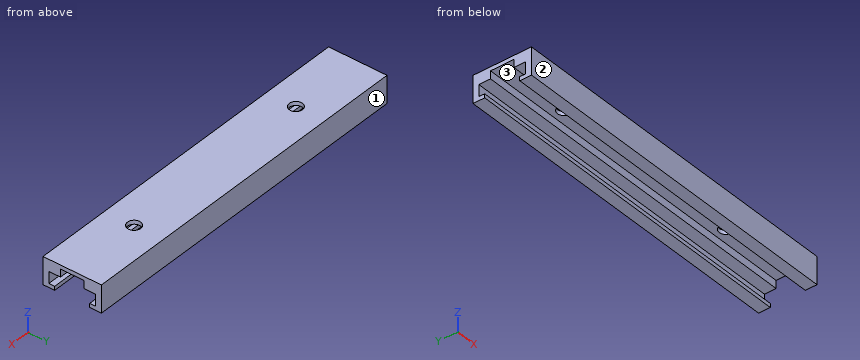
Autodesk Inventor part; units mm, degrees
ref_plane "YZ Plane" through (0, 0, 0) normal (1, 0, 0) x (0, 1, 0)
ref_plane "XZ Plane" through (0, 0, 0) normal (0, 1, 0) x (-1, 0, 0)
ref_plane "XY Plane" through (0, 0, 0) normal (0, 0, 1) x (1, 0, 0)
sketch "スケッチ1" plane through (0, 0, 0) normal (1, 0, 0) x (0, 1, 0)
  line L0 (0, 0) -> (15, 0)
  line L1 (15, 0) -> (15, -7)
  line L2 (0, -7) -> (0, 0)
  line L3 (7.5, 0) -> (7.5, -7)
  line L4 (7.5, -1) -> (10.5, -1)
  line L5 (10.5, -1) -> (10.5, -3)
  line L6 (10.5, -3) -> (13.5, -3)
  line L7 (13.5, -3) -> (13.5, -6)
  line L8 (13.5, -6) -> (12, -6)
  line L9 (12, -6) -> (12, -7)
  line L10 (7.5, -1) -> (4.5, -1)
  line L11 (4.5, -1) -> (4.5, -3)
  line L12 (4.5, -3) -> (1.5, -3)
  line L13 (1.5, -3) -> (1.5, -6)
  line L14 (1.5, -6) -> (3, -6)
  line L15 (3, -6) -> (3, -7)
  line L16 (15, -7) -> (12, -7)
  line L17 (3, -7) -> (0, -7)
  dimension "d0" = 15
  dimension "d1" = 7
  dimension "d2" = 3
  dimension "d3" = 2
  dimension "d5" = 3
  dimension "d6" = 3
  dimension "d7" = 1.5
  dimension "d9" = 1
extrude "押し出し1" add sketch "スケッチ1" along normal blind 90
sketch "スケッチ2" plane through (0, 0, 0) normal (0, 0, 1) x (1, 0, 0)
  line L0 (0, 4.5) -> (0, 10.5)
  line L1 (0, 7.5) -> (90, 7.5)
  line L2 (90, 4.5) -> (90, 10.5)
  line L3 (0, 15) -> (0, 0)
  line L4 (90, 15) -> (90, 0)
  point P0 (19.5, 7.5)
  point P1 (70.5, 7.5)
  dimension "d12" = 19.5
  dimension "d20" = 19.5
hole "穴1" at (19.5, 7.5, 0) at (70.5, 7.5, 0) direction (0, 0, -1) diameter 3.4 end through all
properties part number "slider2a2" material "アルミニウム 6061-AHC"
Could you check a few things on this model? Use its own coordinates, in mm. Face numbers are marked on the shaded views. Give positions to 0.01 mm unless a question says otherwise; leave off trailing zeros. Order: outer loops, then holes, each group sorted by start corner. A loop starts at its lowest first (then second) coordinate and runs counter-clockwise, first axis right, second up. Notation, with made-up numbers: (-17.5, 38.25) - (19.5, 38.25) arc R22 cw to (19.5, 51.25) - close; hole circle Ø5 at (18, -0.5). An arc over 180 degrees is marked (long way). One line per item, written item: value. Start each with the question number.
1. Imagine slicing it at C-C on z = -5.25. List the corners of the cut face in (x, y) for me, plus the area to 3 significant figures.
2. Imagine slicing it at A-A on x = 70.5. List the corners of the cut face in (y, z) for me, plus the area to 3 significant figures.
3. Imagine slicing it at D-D on x = 14.5. List the corners of the cut face in (y, z) for me, plus the area to 3 significant figures.
4. For P1, Ø0.6, axis at x = 51, z = -2.5, coming from the -Y side, with a flat end and sliding along its axis, tell me the tip position at first contact or that it passes through.
5. If I drill on probe 1 along X at (y, z) = (7.5, -0.5); probe 2 along Y at (x, z) = (70, -2.5); probe 3 along Z at (x, y) = (59.5, 13.25), over which ranges is the centre line in solid material (lowest first)?
6. Imagine slicing it at B-B on y = 7.5. List the corners of the cut face in (x, z) for me, plus the area to 3 significant figures.
7. Thinking about a two-plate mould opening in Y: for the marked faces 1, 2 and 3, which applies, +Y half, -Y half, draft (parallel to the pull), parting line (faces both ways), or undercut?
Values:
1. outline: (0, 0) - (90, 0) - (90, 1.5) - (0, 1.5) - close; (0, 13.5) - (90, 13.5) - (90, 15) - (0, 15) - close
1. area: 270 mm²
2. outline: (0, -7) - (3, -7) - (3, -6) - (1.5, -6) - (1.5, -3) - (4.5, -3) - (4.5, -1) - (5.8, -1) - (5.8, 0) - (0, 0) - close; (9.2, -1) - (10.5, -1) - (10.5, -3) - (13.5, -3) - (13.5, -6) - (12, -6) - (12, -7) - (15, -7) - (15, 0) - (9.2, 0) - close
2. area: 44.6 mm²
3. outline: (0, -7) - (3, -7) - (3, -6) - (1.5, -6) - (1.5, -3) - (4.5, -3) - (4.5, -1) - (10.5, -1) - (10.5, -3) - (13.5, -3) - (13.5, -6) - (12, -6) - (12, -7) - (15, -7) - (15, 0) - (0, 0) - close
3. area: 48.0 mm²
4. P1: y = 0
5. probe 1: 0 to 17.8, 21.2 to 68.8, 72.2 to 90
5. probe 2: 0 to 4.5, 10.5 to 15
5. probe 3: -7 to -6, -3 to 0
6. outline: (0, -1) - (17.8, -1) - (17.8, 0) - (0, 0) - close; (21.2, -1) - (68.8, -1) - (68.8, 0) - (21.2, 0) - close; (72.2, -1) - (90, -1) - (90, 0) - (72.2, 0) - close
6. area: 83.2 mm²
7. face 1: +Y half
7. face 2: -Y half
7. face 3: undercut
